from build123d import *
from build123d.topology import SkipClean

# Parameters (mm, degrees)
SKETCH1_W                       = 50
SKETCH1_H                       = 50
BOSS_EXTRUDE1_DEPTH             = 5
BOSS_EXTRUDE3_START             = -25
SKETCH4_W                       = 4
SKETCH4_H                       = 5
BOSS_EXTRUDE3_DEPTH             = 50
CBORE_FOR_M3_SBHCS1_D           = 3.5
CBORE_FOR_M3_SBHCS1_DEPTH       = 10.76
CBORE_FOR_M3_SBHCS1_CBORE_D     = 6.7
CBORE_FOR_M3_SBHCS1_CBORE_DEPTH = 1.65
CBORE_FOR_M3_SBHCS1_TIP         = 1.051506083
CBORE_FOR_M3_SBHCS2_D           = 3
CBORE_FOR_M3_SBHCS2_DEPTH       = 10.76
CBORE_FOR_M3_SBHCS2_CBORE_D     = 6.7
CBORE_FOR_M3_SBHCS2_CBORE_DEPTH = 1.65
CBORE_FOR_M3_SBHCS2_TIP         = 0.901290929
SKETCH19_W                      = 5
SKETCH19_H                      = 20
BOSS_EXTRUDE4_DEPTH             = 20
M5_CLEARANCE_HOLE1_D            = 5.5
FILLET1_R                       = 10
FILLET2_R                       = 5
FILLET3_R                       = 5
FILLET4_R                       = 2.5
FILLET5_R                       = 2.5
SKETCH24_R                      = 4.1
CUT_EXTRUDE1_DEPTH              = 8


# Some blends are built 0.0001 mm under size
with BuildPart() as part:
    # Sketch1 → Boss-Extrude1 (new, symmetric)
    with BuildSketch(Plane(origin=(0, 0, 0), x_dir=(1, 0, 0), z_dir=(0, 1, 0))):
        Rectangle(SKETCH1_W, SKETCH1_H)
    extrude(amount=BOSS_EXTRUDE1_DEPTH, both=True)

    # Sketch4 → Boss-Extrude3 (add)
    with BuildSketch(Plane(origin=(0, 0, 0), x_dir=(0, 0, -1), z_dir=(1, 0, 0)).offset(BOSS_EXTRUDE3_START)):
        with Locations((0, -7.5)):
            Rectangle(SKETCH4_W, SKETCH4_H)
    extrude(amount=BOSS_EXTRUDE3_DEPTH)

    # CBORE for M3 SBHCS1
    with Locations(Plane(origin=(0, -5, 0), x_dir=(-1, 0, 0), z_dir=(0, -1, 0))):
        with Locations((5.656854249, -5.656854249), (-6.717514421, -6.717514421), (6.717514421, 6.717514421), (-5.656854249, 5.656854249)):
            CounterBoreHole(CBORE_FOR_M3_SBHCS1_D / 2, CBORE_FOR_M3_SBHCS1_CBORE_D / 2, CBORE_FOR_M3_SBHCS1_CBORE_DEPTH, depth=CBORE_FOR_M3_SBHCS1_DEPTH)
            with Locations((0, 0, -(CBORE_FOR_M3_SBHCS1_DEPTH + CBORE_FOR_M3_SBHCS1_TIP / 2))):  # 118° drill point
                Cone(0, CBORE_FOR_M3_SBHCS1_D / 2, CBORE_FOR_M3_SBHCS1_TIP, mode=Mode.SUBTRACT)

    # CBORE for M3 SBHCS2
    with Locations(Plane(origin=(0, -5, 0), x_dir=(-1, 0, 0), z_dir=(0, -1, 0))):
        with Locations((17.67766953, 17.67766953), (17.67766953, -17.67766953), (-17.67766953, -17.67766953), (-17.67766953, 17.67766953)):
            CounterBoreHole(CBORE_FOR_M3_SBHCS2_D / 2, CBORE_FOR_M3_SBHCS2_CBORE_D / 2, CBORE_FOR_M3_SBHCS2_CBORE_DEPTH, depth=CBORE_FOR_M3_SBHCS2_DEPTH)
            with Locations((0, 0, -(CBORE_FOR_M3_SBHCS2_DEPTH + CBORE_FOR_M3_SBHCS2_TIP / 2))):  # 118° drill point
                Cone(0, CBORE_FOR_M3_SBHCS2_D / 2, CBORE_FOR_M3_SBHCS2_TIP, mode=Mode.SUBTRACT)

    # Sketch19 → Boss-Extrude4 (add, symmetric)
    with BuildSketch(Plane(origin=(0, 0, 0), x_dir=(0, 0, -1), z_dir=(1, 0, 0))):
        with Locations((12.5, -15)):
            Rectangle(SKETCH19_W, SKETCH19_H)
    boss_extrude4 = extrude(amount=BOSS_EXTRUDE4_DEPTH, both=True)

    # Mirror1: Boss-Extrude4 across plane
    add(boss_extrude4.mirror(Plane.XY))

    # M5 Clearance Hole1 (through all)
    with Locations(Plane.XY.offset(15)):
        with Locations((10, -15)):
            m5_clearance_hole1 = Hole(M5_CLEARANCE_HOLE1_D / 2)

    # Fillet1
    fillet1_edges = [part.edges().sort_by_distance(p)[0] for p in [
        (-25, 0, 25),
        (25, 0, 25),
        (25, 0, -25),
        (-25, 0, -25),
    ]]
    fillet(fillet1_edges, radius=FILLET1_R)

    # Fillet2
    fillet2_edges = [part.edges().sort_by_distance(p)[0] for p in [
        (-20, -25, -12.5),
        (20, -25, -12.5),
        (20, -25, 12.5),
        (-20, -25, 12.5),
    ]]
    fillet(fillet2_edges, radius=FILLET2_R)

    # Fillet3
    fillet3_edges = [part.edges().sort_by_distance(p)[0] for p in [
        (-20, -5, -12.5),
        (20, -5, -12.5),
        (20, -5, 12.5),
        (-20, -5, 12.5),
    ]]
    fillet(fillet3_edges, radius=FILLET3_R - 0.0001)  # a hair under: the kernel refuses the full size

    # Fillet4
    fillet4_edges = [part.edges().sort_by_distance(p)[0] for p in [
        (-25, -10, 0),
        (25, -10, 0),
    ]]
    fillet(fillet4_edges, radius=FILLET4_R)

    # Mirror2: M5 Clearance Hole1 across plane
    add(m5_clearance_hole1.mirror(Plane(origin=(0, 0, 0), x_dir=(0, 0, 1), z_dir=(1, 0, 0))), mode=Mode.SUBTRACT)

    # Fillet5
    # the kernel refuses this fillet: 2.5 mm, written as the material it adds along each edge
    with BuildSketch(Plane(origin=(31.2499, -5, -15), x_dir=(0, 0, -1), z_dir=(-1, 0, 0))) as fillet5_piece_1_section:
        with BuildLine():
            CenterArc((FILLET5_R, FILLET5_R), FILLET5_R, 180, 90)
            Line((0, FILLET5_R), (0, 0))
            Line((0, 0), (FILLET5_R, 0))
        make_face()
    fillet5_piece_1 = extrude(amount=17.809126924, mode=Mode.PRIVATE)
    fillet5_piece_1 = fillet5_piece_1 & Plane(origin=(15, -5.443084519, -15), x_dir=(1, 0, 0), z_dir=(0, 1, 0)) * Cylinder(10, 46, mode=Mode.PRIVATE)
    fillet5_piece_1 = fillet5_piece_1 - Plane(origin=(17.67766953, -5.443084519, -17.67766953), x_dir=(-1, 0, 0), z_dir=(0, -1, 0)) * Cylinder(3.35, 46, mode=Mode.PRIVATE)
    fillet5_piece_1 = fillet5_piece_1 - Plane(origin=(24.9999, -9.9999, -15.600375786), x_dir=(0, 1, 0), z_dir=(0, 0, -1)) * Cylinder(4.9999, 46, mode=Mode.PRIVATE)
    add(fillet5_piece_1)
    with BuildSketch(Plane(origin=(-21.914565984, -5, -15), x_dir=(0, 0, -1), z_dir=(1, 0, 0))) as fillet5_piece_2_section:
        with BuildLine():
            CenterArc((FILLET5_R, -FILLET5_R), FILLET5_R, 90, 90)
            Line((0, -FILLET5_R), (0, 0))
            Line((0, 0), (FILLET5_R, 0))
        make_face()
    fillet5_piece_2 = extrude(amount=43.829131967, mode=Mode.PRIVATE)
    fillet5_piece_2 = fillet5_piece_2 - Plane(origin=(-24.9999, -9.9999, -15.47958938), x_dir=(0, 1, 0), z_dir=(0, 0, -1)) * Cylinder(4.9999, 98, mode=Mode.PRIVATE)
    fillet5_piece_2 = fillet5_piece_2 - Plane(origin=(-17.67766953, -5.581152755, -17.67766953), x_dir=(-1, 0, 0), z_dir=(0, -1, 0)) * Cylinder(3.35, 98, mode=Mode.PRIVATE)
    fillet5_piece_2 = fillet5_piece_2 - Plane(origin=(17.67766953, -5.581152755, -17.67766953), x_dir=(-1, 0, 0), z_dir=(0, -1, 0)) * Cylinder(3.35, 98, mode=Mode.PRIVATE)
    fillet5_piece_2 = fillet5_piece_2 - Plane(origin=(24.9999, -9.9999, -15.47958938), x_dir=(0, 1, 0), z_dir=(0, 0, -1)) * Cylinder(4.9999, 98, mode=Mode.PRIVATE)
    add(fillet5_piece_2)
    with BuildSketch(Plane(origin=(-13.440773076, -5, -15), x_dir=(0, 0, -1), z_dir=(-1, 0, 0))) as fillet5_piece_3_section:
        with BuildLine():
            CenterArc((FILLET5_R, FILLET5_R), FILLET5_R, 180, 90)
            Line((0, FILLET5_R), (0, 0))
            Line((0, 0), (FILLET5_R, 0))
        make_face()
    fillet5_piece_3 = extrude(amount=17.809126924, mode=Mode.PRIVATE)
    fillet5_piece_3 = fillet5_piece_3 & Plane(origin=(-15, -5.616758161, -15), x_dir=(-1, 0, 0), z_dir=(0, -1, 0)) * Cylinder(10, 46, mode=Mode.PRIVATE)
    fillet5_piece_3 = fillet5_piece_3 - Plane(origin=(-24.9999, -9.9999, -15.466172453), x_dir=(0, 1, 0), z_dir=(0, 0, -1)) * Cylinder(4.9999, 46, mode=Mode.PRIVATE)
    fillet5_piece_3 = fillet5_piece_3 - Plane(origin=(-17.67766953, -5.616758161, -17.67766953), x_dir=(-1, 0, 0), z_dir=(0, -1, 0)) * Cylinder(3.35, 46, mode=Mode.PRIVATE)
    add(fillet5_piece_3)
    with BuildSketch(Plane(origin=(31.2499, -5, 15), x_dir=(0, 0, 1), z_dir=(-1, 0, 0))) as fillet5_piece_4_section:
        with BuildLine():
            CenterArc((FILLET5_R, -FILLET5_R), FILLET5_R, 90, 90)
            Line((0, -FILLET5_R), (0, 0))
            Line((0, 0), (FILLET5_R, 0))
        make_face()
    fillet5_piece_4 = extrude(amount=17.809126924, mode=Mode.PRIVATE)
    fillet5_piece_4 = fillet5_piece_4 & Plane(origin=(15, -5.443086439, 15), x_dir=(0, 0, 1), z_dir=(0, 1, 0)) * Cylinder(10, 46, mode=Mode.PRIVATE)
    fillet5_piece_4 = fillet5_piece_4 - Plane(origin=(24.9999, -9.9999, 15.600377701), x_dir=(0, 1, 0), z_dir=(0, 0, 1)) * Cylinder(4.9999, 46, mode=Mode.PRIVATE)
    fillet5_piece_4 = fillet5_piece_4 - Plane(origin=(17.67766953, -5.443086439, 17.67766953), x_dir=(-1, 0, 0), z_dir=(0, -1, 0)) * Cylinder(3.35, 46, mode=Mode.PRIVATE)
    add(fillet5_piece_4)
    with BuildSketch(Plane(origin=(-21.914565984, -5, 15), x_dir=(0, 0, 1), z_dir=(1, 0, 0))) as fillet5_piece_5_section:
        with BuildLine():
            CenterArc((FILLET5_R, FILLET5_R), FILLET5_R, 180, 90)
            Line((0, FILLET5_R), (0, 0))
            Line((0, 0), (FILLET5_R, 0))
        make_face()
    fillet5_piece_5 = extrude(amount=43.829131967, mode=Mode.PRIVATE)
    fillet5_piece_5 = fillet5_piece_5 - Plane(origin=(24.9999, -9.9999, 15.479588149), x_dir=(0, 1, 0), z_dir=(0, 0, 1)) * Cylinder(4.9999, 98, mode=Mode.PRIVATE)
    fillet5_piece_5 = fillet5_piece_5 - Plane(origin=(17.67766953, -5.581152089, 17.67766953), x_dir=(-1, 0, 0), z_dir=(0, -1, 0)) * Cylinder(3.35, 98, mode=Mode.PRIVATE)
    fillet5_piece_5 = fillet5_piece_5 - Plane(origin=(-17.67766953, -5.581152089, 17.67766953), x_dir=(-1, 0, 0), z_dir=(0, -1, 0)) * Cylinder(3.35, 98, mode=Mode.PRIVATE)
    fillet5_piece_5 = fillet5_piece_5 - Plane(origin=(-24.9999, -9.9999, 15.479588149), x_dir=(1, 0, 0), z_dir=(0, 0, 1)) * Cylinder(4.9999, 98, mode=Mode.PRIVATE)
    add(fillet5_piece_5)
    with BuildSketch(Plane(origin=(-13.440773076, -5, 15), x_dir=(0, 0, 1), z_dir=(-1, 0, 0))) as fillet5_piece_6_section:
        with BuildLine():
            CenterArc((FILLET5_R, -FILLET5_R), FILLET5_R, 90, 90)
            Line((0, -FILLET5_R), (0, 0))
            Line((0, 0), (FILLET5_R, 0))
        make_face()
    fillet5_piece_6 = extrude(amount=17.809126924, mode=Mode.PRIVATE)
    fillet5_piece_6 = fillet5_piece_6 & Plane(origin=(-15, -5.616758645, 15), x_dir=(0, 0, 1), z_dir=(0, -1, 0)) * Cylinder(10, 46, mode=Mode.PRIVATE)
    fillet5_piece_6 = fillet5_piece_6 - Plane(origin=(-17.67766953, -5.616758645, 17.67766953), x_dir=(-1, 0, 0), z_dir=(0, -1, 0)) * Cylinder(3.35, 46, mode=Mode.PRIVATE)
    fillet5_piece_6 = fillet5_piece_6 - Plane(origin=(-24.9999, -9.9999, 15.466173234), x_dir=(1, 0, 0), z_dir=(0, 0, 1)) * Cylinder(4.9999, 46, mode=Mode.PRIVATE)
    add(fillet5_piece_6)

    # Sketch24 → Cut-Extrude1 (cut)
    with SkipClean():  # the faces are left unmerged after this step: merging them gives an invalid solid
        with BuildSketch(Plane(origin=(0, 5, 0), x_dir=(1, 0, 0), z_dir=(0, 1, 0))):
            with Locations(Location((0, 0, 0), (0, 0, 270))):
                Circle(SKETCH24_R)
        extrude(amount=-CUT_EXTRUDE1_DEPTH, mode=Mode.SUBTRACT)
    add(part.part.scale(1), mode=Mode.REPLACE)  # the faces are merged on a copy


solid = part.part
For this review, take the finished solid that the model builds, in its own axes (mm). A direction names the side the tool comes from. Give positions to 0.01 mm unless a question says otherwise; leave off trailing zeros. Loops run counter-clockwise (first coordinate to the right, second up) from the corner with the lowest first, then second, coordinate; pieces in that order, holes last. Notation, with made-up numbers: M -16,51.5 L -7,51.5 A31 ccw -7,75.5 Z; hole C -8.5,35 d3. An arc over 180 degrees is marked long. Answer as a JSON object with one key per item and string values. Group by question number.
Q1. For probe 1 along Z at (x, y) = (-18.5, -7); probe 2 along Z at (x, y) = (1, -16.5); probe 3 along Y at (x, z) = (14, 0), list the stretches that pass through material, from the lowest coordinate up. Write a range as [from, to].
Q2. Tool access review of faces 1 (the flat face through (20, -15, -12)), 2 (the cylindrical face through (-21, -7, 13)), 3 (the flat face through (-20, -15, -12)): name each direction out of +Z, -Z, +X, -X, +Y, -Y from which nothing blocks a thin tool from reaching the whole face with its end or side.
Q3. Insertion check: P1, Ø1, axis at y = -11.5, z = -3.5, coming from the +X side; P2, Ø7, axis at x = -10, y = -15, coming from the -Z side; P3, Ø6, axis at x = -11, z = 20.5, coming from the -Y side; P4, Ø5.5, axis at x = -7, y = -8, coming from the +Z side. Each pin has a flat end and moves straight along its axis. Give the tip position at first contact, or say it passes through.
Q4. Add section B-B on z = -13.5. Give the number of separate pieces and of enclosed holes in the cut face, and give its area (3 significant figures).
Q5. Add section A-A on y = -15. Give the boundary of the cut face in (x, z), and give its area (3 significant figures).
Q6. Add section D-D on x = 0. Give the boundary of the cut face in (y, z), and give its area (3 significant figures).
Q7. Mouldability with a two-part tool opening along Z and no side actions: class faces 4 (the cylindrical face through (24.248, -9.287, -0.028)), 5 (the cylindrical face through (-15.02, -4.53, -15.64)), 6 (the cylindrical face through (-22.15, 0.07, 21.99)), 7 (the flat face through (-16, -3.35, 18)) as +Z half, -Z half, draft (parallel to the pull), parting line (faces both ways), or undercut.
Q8. Add section C-C on y = -21. Give the boundary of the cut face in (x, z).
Checked values:
{
 "1": {"probe 1": "[-15, -10], [-2, 2], [10, 15]", "probe 2": "[-15, -10], [10, 15]", "probe 3": "[-10, 5]"},
 "2": {"face 1": "+Z, -Z, +X, -Y", "face 2": "+Z, -X, -Y", "face 3": "+Z, -Z, -X, -Y"},
 "3": {"P1": "through", "P2": "z = -15", "P3": "y = -5", "P4": "z = 16.41"},
 "4": {"separate pieces": "1", "enclosed holes": "2", "area": "1,250 mm²"},
 "5": {"outline": "M -20,-15 L -12.75,-15 L -12.75,-10 L -20,-10 Z; M -20,10 L -12.75,10 L -12.75,15 L -20,15 Z; M -7.25,-15 L 7.25,-15 L 7.25,-10 L -7.25,-10 Z; M -7.25,10 L 7.25,10 L 7.25,15 L -7.25,15 Z; M 12.75,-15 L 20,-15 L 20,-10 L 12.75,-10 Z; M 12.75,10 L 20,10 L 20,15 L 12.75,15 Z", "area": "290 mm²"},
 "6": {"outline": "M -25,-15 L -7.5,-15 A2.5 cw -5,-17.5 L -5,-25 L 5,-25 L 5,-4.1 L -3,-4.1 L -3,4.1 L 5,4.1 L 5,25 L -5,25 L -5,17.5 A2.5 cw -7.5,15 L -25,15 L -25,10 L -5,10 L -5,2 L -10,2 L -10,-2 L -5,-2 L -5,-10 L -25,-10 Z", "area": "657 mm²"},
 "7": {"face 4": "draft", "face 5": "undercut", "face 6": "+Z half", "face 7": "undercut"},
 "8": {"outline": "M -19.9,-15 L 19.9,-15 L 19.9,-10 L -19.9,-10 Z; M -19.9,10 L 19.9,10 L 19.9,15 L -19.9,15 Z"}
}
